For this review, take the finished solid that the model builds, in its own axes (mm). A direction names the side the tool comes from. Round coordinates to 2 decimals unless told otherwise and drop trailing zeros. Loops run counter-clockwise (first coordinate to the right, second up) from the corner with the lowest first, then second, coordinate; pieces in that order, holes last.
1. Draft analysis for pull direction X (two halves, no side actions). For faces 3 (the flat face through (36.01, -0.03, -28)), 4 (the cylindrical face through (47.878, 0.028, -7.795)), 5 (the cylindrical face through (0.07, -0.03, -12.6)), state which applies: released by +X, released by -X, zero draft, split by the parting line, or undercut.
2. To check wall thickness, follow line 1 along X through (y, z) = (0.9, -37); line 2 along X through (y, z) = (0.75, 11); line 3 along X through (y, z) = (1.25, -26). State the ranges of each line that lie inside material, in increasing order.
3. Consider section D-D on x = 20. State the section outline as (y, z) points, then the cut area to 3 significant figures.
4. Tool access review of faces 1 (the cylindrical face through (6.05, 0.03, 11.07)), 2 (the flat face through (21.522, -0.028, -10.594)): name each direction out of +Z, -Z, +X, -X, +Y, -Y from which nothing blocks a thin tool from reaching the whole face with its end or side.
5. Consider section A-A on x = 0. State the section outline as (y, z) points, then the cut area to 3 significant figures.
6. Consider section B-B on x = 42. State the section outline as (y, z) points.
7. Consider section C-C on y = 1. State how many separate pieces and enclosed holes the cut face has, then the cut area to 3 significant figures.
8. Clearance check with flat-ended pins moving along their axes: pin 1 Ø1 at (y, z) = (-1, -15.5) entering from -X; pin 2 Ø1 at (x, y) = (24.5, 1) entering from +Z. State where each tip first meets the part, or that it passes through.
from build123d import *

# Parameters (mm, degrees)
BOSS_EXTRUDE1_DEPTH      = 2
BOSS_EXTRUDE1_DEPTH_BACK = 2
SKETCH1_R                = 1.6
BOSS_EXTRUDE3_DEPTH      = 2
BOSS_EXTRUDE3_DEPTH_BACK = 2
SKETCH3_R                = 1.55
FILLET1_R                = 7


with BuildPart() as part:
    # Sketch1 → Boss-Extrude1 (new, two sides: drawn at the far end of the back side and taken through both)
    with BuildSketch(Plane(origin=(0, 0, 0), x_dir=(1, 0, 0), z_dir=(0, 1, 0)).offset(-BOSS_EXTRUDE1_DEPTH_BACK)):
        with BuildLine():
            ThreePointArc((5, 11), (0, 16), (-5, 11))
            Line((-5, 11), (-5, -11))
            ThreePointArc((-5, -11), (0, -16), (5, -11))
            Line((5, -11), (5, 11))
        make_face()
        with Locations(Location((0, 11, 0), (0, 0, 270))):
            Circle(SKETCH1_R, mode=Mode.SUBTRACT)
        with Locations(Location((0, -11, 0), (0, 0, 270))):
            Circle(SKETCH1_R, mode=Mode.SUBTRACT)
    extrude(amount=BOSS_EXTRUDE1_DEPTH + BOSS_EXTRUDE1_DEPTH_BACK)

    # Sketch3 → Boss-Extrude3 (add, two sides: drawn at the far end of the back side and taken through both)
    with BuildSketch(Plane(origin=(0, 0, 0), x_dir=(1, 0, 0), z_dir=(0, 1, 0)).offset(-BOSS_EXTRUDE3_DEPTH_BACK)):
        with BuildLine():
            Line((34.468399727, 13.95420099), (5, 6.305712988))
            Line((5, 6.305712988), (5, -11))
            Line((5, -11), (49.334489528, 6.966618691))
            Line((49.334489528, 6.966618691), (47, 37))
            ThreePointArc((47, 37), (42, 42), (37, 37))
            Line((37, 37), (34.468399727, 13.95420099))
        make_face()
        with Locations(Location((42, 37, 0), (0, 0, 270))):
            Circle(SKETCH3_R, mode=Mode.SUBTRACT)
    extrude(amount=BOSS_EXTRUDE3_DEPTH + BOSS_EXTRUDE3_DEPTH_BACK)

    # Fillet1
    fillet1_edges = [part.edges().sort_by_distance(p)[0] for p in [
        (5, 0, 11),
        (49.334489528, 0, -6.966618691),
        (34.468399727, 0, -13.95420099),
        (5, 0, -6.305712988),
    ]]
    fillet(fillet1_edges, radius=FILLET1_R)


solid = part.part
Resolved:
1. face 3: released by -X
1. face 4: released by +X
1. face 5: undercut
2. line 1: x = 37 to 40.45, 43.55 to 47
2. line 2: x = -5 to -1.6, 1.6 to 6.13
2. line 3: x = 35.79 to 47.86
3. outline: (-2, -10.2) - (2, -10.2) - (2, 4.92) - (-2, 4.92) - close
3. area: 60.5 mm2
4. face 1: +Z, +X, +Y, -Y
4. face 2: -Z, +Y, -Y
5. outline: (-2, -16) - (2, -16) - (2, -12.6) - (-2, -12.6) - close; (-2, -9.4) - (2, -9.4) - (2, 9.4) - (-2, 9.4) - close; (-2, 12.6) - (2, 12.6) - (2, 16) - (-2, 16) - close
5. area: 102 mm2
6. outline: (-2, -42) - (2, -42) - (2, -38.55) - (-2, -38.55) - close; (-2, -35.45) - (2, -35.45) - (2, -3.99) - (-2, -3.99) - close
7. separate pieces: 1
7. enclosed holes: 3
7. area: 1,200 mm2
8. pin 1: stops at x = -3
8. pin 2: stops at z = 3.3
